from build123d import *

# Parameters (mm, degrees)
SKETCH1_W           = 36.322
SKETCH1_H           = 16.256
BOSS_EXTRUDE1_DEPTH = 4.953
SKETCH2_R           = 2.54
BOSS_EXTRUDE2_DEPTH = 17.78
FILLET1_R           = 2.54
FILLET2_R           = 2.54
FILLET3_R           = 1.27


with BuildPart() as part:
    # Sketch1 → Boss-Extrude1 (new body)
    with BuildSketch(Plane(origin=(0, 0, 0), x_dir=(1, 0, 0), z_dir=(0, 1, 0))):
        with Locations((18.161, -8.128)):
            Rectangle(SKETCH1_W, SKETCH1_H)
    extrude(amount=BOSS_EXTRUDE1_DEPTH)

    # Sketch2 → Boss-Extrude2 (add)
    with BuildSketch(Plane(origin=(0, 4.953, 0), x_dir=(1, 0, 0), z_dir=(0, 1, 0))):
        with Locations(Location((18.161, -8.128, 0), (0, 0, 270))):
            Circle(SKETCH2_R)
    extrude(amount=BOSS_EXTRUDE2_DEPTH)

    # Fillet1
    fillet1_edges = [part.edges().sort_by_distance(p)[0] for p in [
        (18.161, 22.733, 5.588),
    ]]
    fillet(fillet1_edges, radius=FILLET1_R)

    # Fillet2
    fillet2_edges = [part.edges().sort_by_distance(p)[0] for p in [
        (18.161, 4.953, 5.588),
    ]]
    fillet(fillet2_edges, radius=FILLET2_R)

    # Fillet3
    fillet3_edges = [part.edges().sort_by_distance(p)[0] for p in [
        (0, 2.4765, 0),
        (36.322, 2.4765, 0),
        (36.322, 2.4765, 16.256),
        (0, 2.4765, 16.256),
    ]]
    fillet(fillet3_edges, radius=FILLET3_R)


solid = part.part
CAD build for the part. Positions are in the model's coordinates, mm. A direction names the side the tool comes from. Give positions to 0.01 mm unless a question says otherwise; leave off trailing zeros. Write each loop counter-clockwise with the first axis right and the second up, starting at its lowest first coordinate (ties: lowest second). Pieces come first, ordered by that corner, then holes. Notation, with made-up numbers: (58, 53.25) - (108, 53.25) arc R27 cw to (108, 73.25) - close; hole circle Ø6 at (81.5, 1). An arc over 180 degrees is marked (long way). Put each result on its own line as item: value.
(1) Wall check: L1, parallel to Y at x = 25, z = 8.5; L2, parallel to X at y = 8, z = 10.25; L3, parallel to Z at x = 18, y = 20.75. Give the ranges that are in metal, low to high.
Working result:
L1: 0 to 4.95
L2: 16.77 to 19.56
L3: 5.66 to 10.6
(2) Saw through at B-B (y = 17.75). List the corners of the cut face in (x, z).
Working result:
outline: circle Ø5.08 at (18.16, 8.13)
(3) Drop flat-ended pins along their axis: pin 1 Ø8 at (y, z) = (8.5, 13) entering from +X; pin 2 Ø5 at (y, z) = (13.5, 10) entering from -X; pin 3 Ø8 at (x, y) = (17, 18.5) entering from +Z. Give the stop position or say it passes through.
Working result:
pin 1: x = 36.32
pin 2: x = 15.62
pin 3: z = 10.67
(4) Saw through at A-A (x = 30). List the corners of the cut face in (y, z), then the cut area to 3 significant figures.
Working result:
outline: (0, 0) - (4.95, 0) - (4.95, 16.26) - (0, 16.26) - close
area: 80.5 mm^2
(5) Pull direction Y, two halves, no side cores. Call faces 1 (the cylindrical face through (35.94, 2.51, 0.36)), 2 (the flat face through (14, 4.953, 12)), 3 (the flat face through (18, 0, 8)): released by +Y, released by -Y, zero draft, split by the parting line, or undercut.
Working result:
face 1: zero draft
face 2: released by +Y
face 3: released by -Y
(6) Tool access for faces 4 (the cylindrical face through (20.3, 13.8, 9.5)), 5 (the cylindrical face through (35.94, 2.511, 15.894)): list every direction of +Z, -Z, +X, -X, +Y, -Y with a clear straight run to the whole face (end or side of a thin tool).
Working result:
face 4: +Y
face 5: +Z, +X, +Y, -Y
